from build123d import *

# Parameters (mm, degrees)
SKETCH1_R               = 15.24
BOSS_EXTRUDE1_DEPTH     = 17.526
CUT_EXTRUDE2_DEPTH      = 33.139783384
BOSS_EXTRUDE2_DEPTH     = 38.1
CUT_EXTRUDE1_DEPTH      = 35.33136764
CUT_EXTRUDE1_DEPTH_BACK = 35.33136764
SKETCH4_W               = 17.018
SKETCH4_H               = 6.35
SKETCH4_W_2             = 5.461
FILLET1_R               = 0.254
FILLET2_R               = 1.016


with BuildPart() as part:
    # Sketch1 → Boss-Extrude1 (new body)
    with BuildSketch(Plane.XY):
        with BuildLine():
            Line((-19.05, 0), (-19.05, -16.002))
            Line((-19.05, -16.002), (19.05, -16.002))
            Line((19.05, -16.002), (19.05, 0))
            ThreePointArc((19.05, 0), (0, 19.05), (-19.05, 0))
        make_face()
        Circle(SKETCH1_R, mode=Mode.SUBTRACT)
    extrude(amount=BOSS_EXTRUDE1_DEPTH)

    # Sketch5 → Cut-Extrude2 (cut, through all)
    with BuildSketch(Plane.XY.offset(17.526)):
        with BuildLine():
            Line((19.05, -5.474194202), (19.05, 0))
            ThreePointArc((19.05, 0), (18.848061086, 2.766422474), (18.246525637, 5.474194202))
            Line((18.246525637, 5.474194202), (14.222896957, 5.474194202))
            ThreePointArc((14.222896957, 5.474194202), (15.24, 0), (14.222896957, -5.474194202))
            Line((14.222896957, -5.474194202), (19.05, -5.474194202))
        make_face()
    extrude(amount=-CUT_EXTRUDE2_DEPTH, mode=Mode.SUBTRACT)

    # Sketch3 → Boss-Extrude2 (add)
    with BuildSketch(Plane(origin=(19.05, 0, 0), x_dir=(0, 0, -1), z_dir=(1, 0, 0))):
        Polygon((-2.794, -16.002), (-2.794, -22.352), (0.254, -22.352), (-0.254, -16.002), align=None)
        Polygon((-14.732, -16.002), (-14.732, -22.352), (-17.78, -22.352), (-17.272, -16.002), align=None)
    extrude(amount=-BOSS_EXTRUDE2_DEPTH)

    # Sketch4 → Cut-Extrude1 (cut, two sides: drawn at the far end of the back side and taken through both)
    with BuildSketch(Plane(origin=(0, 0, 0), x_dir=(-1, 0, 0), z_dir=(0, 0, -1)).offset(-CUT_EXTRUDE1_DEPTH_BACK)):
        with Locations((0, -19.177)):
            Rectangle(SKETCH4_W, SKETCH4_H)
        with Locations((16.3195, -19.177)):
            Rectangle(SKETCH4_W_2, SKETCH4_H)
        with Locations((-16.3195, -19.177)):
            Rectangle(SKETCH4_W_2, SKETCH4_H)
    extrude(amount=CUT_EXTRUDE1_DEPTH + CUT_EXTRUDE1_DEPTH_BACK, mode=Mode.SUBTRACT)

    # Fillet1
    fillet1_edges = [part.edges().sort_by_distance(p)[0] for p in [
        (13.589, -19.177, 14.732),
        (13.589, -22.352, 1.27),
        (13.589, -22.352, 16.256),
        (-13.589, -19.177, 0),
        (-13.589, -19.177, 2.794),
        (-13.589, -19.177, 14.732),
        (-13.589, -22.352, 1.27),
        (-13.589, -22.352, 16.256),
        (8.509, -19.177, 0),
        (8.509, -19.177, 2.794),
        (8.509, -19.177, 14.732),
        (8.509, -22.352, 1.27),
        (-8.509, -19.177, 0),
        (-8.509, -19.177, 2.794),
        (-8.509, -19.177, 14.732),
        (-8.509, -22.352, 1.27),
        (8.509, -22.352, 16.256),
        (-8.509, -22.352, 16.256),
        (-11.049, -22.352, 17.78),
        (11.049, -22.352, 17.78),
        (-8.509, -19.177, 17.526),
        (8.509, -19.177, 17.526),
        (-13.589, -19.177, 17.526),
        (13.589, -19.177, 17.526),
        (-11.049, -22.352, 14.732),
        (11.049, -22.352, 14.732),
        (-11.049, -22.352, 2.794),
        (11.049, -22.352, 2.794),
        (-11.049, -22.352, -0.254),
        (11.049, -22.352, -0.254),
        (13.589, -19.177, 0),
        (13.589, -19.177, 2.794),
    ]]
    fillet(fillet1_edges, radius=FILLET1_R)

    # Fillet2
    fillet2_edges = [part.edges().sort_by_distance(p)[0] for p in [
        (18.246525637, 5.474194202, 8.763),
        (19.05, -5.474194202, 8.763),
        (14.222896957, -5.474194202, 8.763),
        (14.222896957, 5.474194202, 8.763),
    ]]
    fillet(fillet2_edges, radius=FILLET2_R)


solid = part.part
Verification items for the finished model (mm, model axes). A direction names the side the tool comes from. Round coordinates to 2 decimals unless told otherwise and drop trailing zeros. Loops run counter-clockwise (first coordinate to the right, second up) from the corner with the lowest first, then second, coordinate; pieces in that order, holes last. Notation, with made-up numbers: (78.5, 48.25) - (128.5, 48.25) arc R29 ccw to (128.5, 87.25) - close; hole circle Ø1 at (88.25, -21.5). An arc over 180 degrees is marked (long way). Answer in a Markdown table with one row per item. Add a question column.
Q1. Release check for a two-part mould opening along Y. For faces 1 (the face through (-11, -22.352, 1)), 2 (the face through (11.081, -19.082, 0.008)), 3 (the face through (13.589, -19, 1)) record: pulls with the +Y half, pulls with the -Y half, needs draft (parallel to the pull), parting line crosses it, or undercut.
Q2. Tool access check on faces 4 (the face through (-8.509, -19, 16)), 5 (the face through (11, -19, 14.732)), 6 (the face through (-16, -1, 17.526)), 7 (the face through (-16, -1, 0)). Record the directions out of +Z, -Z, +X, -X, +Y, -Y that give a thin tool (end or side, any length) a straight path to the whole face; none if there is none.
Q3. Section check B-B on z = 7. Enter the section's corners in (x, y).
Q4. Section check C-C on y = 13.5. Enter the section's corners in (x, z).
Q5. Section check A-A on x = 0. Enter the section's corners in (y, z), plus the area to 3 significant figures.
Q6. Material ranges on line 1 (Y direction, x = 0, z = 7.75); line 2 (Z direction, x = -12.5, y = -11); line 3 (X direction, y = 0, z = 10.75), recorded low to high.
Q7. Gauge pin test, flat ends, axial feed: pin 1 (2 mm diameter, centred on y = -19, z = 16, fed in from +X); pin 2 (1.4 mm diameter, centred on x = 11.5, y = -19, fed in from +Z); pin 3 (3.5 mm diameter, centred on x = -11.5, y = -19.5, fed in from +Z). Record the tip position at first contact, or that the pin passes through.
Q8. Section check D-D on x = -12. Enter the section's corners in (y, z).
Found:
| question | item | result |
|---|---|---|
| 1 | face 1 | pulls with the -Y half |
| 1 | face 2 | undercut |
| 1 | face 3 | needs draft |
| 2 | face 4 | +Z, -Z, -Y |
| 2 | face 5 | +X, -X, -Y |
| 2 | face 6 | +Z, +X, -X, +Y |
| 2 | face 7 | -Z, +X, -X, +Y |
| 3 | outline | (-19.05, -16) - (19.05, -16) - (19.05, -6.49) arc R1.02 ccw to (18.03, -5.47) - (14.9, -5.47) arc R1.02 ccw to (13.97, -6.08) arc R15.24 cw (long way) to (13.97, 6.08) arc R1.02 ccw to (14.9, 5.47) - (16.83, 5.47) arc R1.02 ccw to (17.77, 6.86) arc R19.05 ccw to (-19.05, 0) - close |
| 4 | outline | (-13.44, 0) - (-7.07, 0) - (-7.07, 17.53) - (-13.44, 17.53) - close; (7.07, 0) - (13.44, 0) - (13.44, 17.53) - (7.07, 17.53) - close |
| 5 | outline | (-16, 0) - (-15.24, 0) - (-15.24, 17.53) - (-16, 17.53) - close; (15.24, 0) - (19.05, 0) - (19.05, 17.53) - (15.24, 17.53) - close |
| 5 | area | 80.1 mm² |
| 6 | line 1 | y = -16 to -15.24, 15.24 to 19.05 |
| 6 | line 2 | z = 0 to 17.53 |
| 6 | line 3 | x = -19.05 to -15.24 |
| 7 | pin 1 | stops at x = 13.59 |
| 7 | pin 2 | stops at z = 17.57 |
| 7 | pin 3 | stops at z = 17.69 |
| 8 | outline | (-22.35, 0.02) arc R0.25 ccw to (-22.08, -0.23) - (-16, 0.25) - (-16, 0) - (-9.39, 0) - (-9.39, 17.53) - (-16, 17.53) - (-16, 17.27) - (-22.08, 17.76) arc R0.25 ccw to (-22.35, 17.5) - (-22.35, 14.99) arc R0.25 ccw to (-22.1, 14.73) - (-16, 14.73) - (-16, 2.79) - (-22.1, 2.79) arc R0.25 ccw to (-22.35, 2.54) - close; (9.39, 0) - (14.8, 0) - (14.8, 17.53) - (9.39, 17.53) - close |
